Can you work these out from the model? Positions are in its coordinate system, mm. Face numbers are marked on the shaded views. A direction names the side the tool comes from. Give positions to 0.01 mm unless a question says otherwise; leave off trailing zeros. Order: outer loops, then holes, each group sorted by start corner. A loop starts at its lowest first (then second) coordinate and runs counter-clockwise, first axis right, second up.
Item 1: I want a section at D-D, the plane x = 125.5. Write out the boundary of the cut face in (y, z).
Item 2: I want a section at A-A, the plane y = -15. Write out the boundary of the cut face in (x, z).
Item 3: I'm going to push flat-ended pins straight in: pin 1 Ø8 at (x, y) = (112.5, 13.5) entering from +Z; pin 2 Ø10.5 at (x, z) = (144, 12) entering from +Y; pin 3 Ø1.5 at (y, z) = (-18, 6) entering from +X. Where does each tip first touch, or does it pass through?
Item 4: If we mould it in two halves opening along X, with no side actions, what happens to the marked faces 6, 7 and 8? For each: +X half, -X half, draft (parallel to the pull), parting line (faces both ways), or undercut.
Item 5: Which directions (+Z, -Z, +X, -X, +Y, -Y) give clear straight access to the entire face, cutting with the end or side of a thin tool? Please do the marked faces 1, 2, 3, 4 and 5.
Item 6: If I drill on line 1 along Y through (x, z) = (-1.5, -19); line 2 along Z through (x, y) = (0, 17.75); line 3 along X through (y, z) = (15.5, 10.5), over which ranges is the centre line in solid material (lowest first)?
Item 7: I want a section at B-B, the plane x = 2. Write out the boundary of the cut face in (y, z), then the cut area to 3 significant figures.
Item 8: I want a section at C-C, the plane y = 18.5. Write out the boundary of the cut face in (x, z), then the cut area to 3 significant figures.
```python
from build123d import *

# Parameters (mm, degrees)
F1_DEPTH      = 30.1625
F1_DEPTH_BACK = 30.1625
F2_DEPTH      = 11.1125
F2_DEPTH_BACK = 30.1625
F0_R          = 12.7
F3_DEPTH      = 30.1625
F3_DEPTH_BACK = 30.1625
F4_W          = 41.275
F4_H          = 34.798
F5_DEPTH      = 38.1
F6_W          = 11.1633
F6_H          = 50.8
F7_DEPTH      = 25.4
F7_DEPTH_BACK = 25.4
F8_R          = 6.35
F9_DEPTH      = 25.4
F10_R         = 7.874
F11_R         = 5.08
F12_F1_R      = 3.302
F12_F2_R      = 3.302


with BuildPart() as f1:
    # F0 (on Front) → F1 (new body, two sides)
    with BuildSketch(Plane.XZ) as f1_sk:
        with BuildLine():
            ThreePointArc((131.0386, 34.798), (127.4644153616, 16.0823576341), (117.2464, 0))
            Line((117.2464, 0), (117.2464, -22.352))
            Line((117.2464, -22.352), (194.2084, -22.352))
            Line((194.2084, -22.352), (194.2084, 0))
            Line((194.2084, 0), (150.0886, 0))
            Line((150.0886, 0), (150.0886, 34.798))
            Line((150.0886, 34.798), (131.0386, 34.798))
        make_face()
    extrude(amount=-F1_DEPTH)
    extrude(f1_sk.sketch, amount=F1_DEPTH_BACK)

    # F0 (on Front) → F2 (join, two sides)
    with BuildSketch(Plane.XZ) as f2_sk:
        Polygon((117.2464, 0), (85.852, 0), (91.8464, -22.352), (117.2464, -22.352), align=None)
    extrude(amount=F2_DEPTH)
    extrude(f2_sk.sketch, amount=-F2_DEPTH_BACK)

    # F0 (on Front) → F3 (join, two sides)
    with BuildSketch(Plane.XZ) as f3_sk:
        with BuildLine():
            Line((85.852, 0), (22.352, 0))
            ThreePointArc((22.352, 0), (15.8052507731, -15.8052507731), (0, -22.352))
            Line((0, -22.352), (91.8464, -22.352))
            Line((91.8464, -22.352), (85.852, 0))
        make_face()
        with BuildLine():
            ThreePointArc((0, -22.352), (15.8052507731, -15.8052507731), (22.352, 0))
            ThreePointArc((22.352, 0), (-15.8052507731, 15.8052507731), (0, -22.352))
        make_face()
        Circle(F0_R, mode=Mode.SUBTRACT)
    extrude(amount=F3_DEPTH)
    extrude(f3_sk.sketch, amount=-F3_DEPTH_BACK)

    # F4 (on face) → F5 (cut)
    with BuildSketch(Plane.YZ.offset(150.0886)):
        with Locations((9.525, 17.399)):
            Rectangle(F4_W, F4_H)
    extrude(amount=-F5_DEPTH, mode=Mode.SUBTRACT)

    # F6 (on Right) → F7 (cut, two sides)
    with BuildSketch(Plane.YZ) as f7_sk:
        with Locations((5.58165, 25.4)):
            Rectangle(F6_W, F6_H)
        with Locations((-5.58165, 25.4)):
            Rectangle(F6_W, F6_H)
        Polygon((11.1633, 0), (0, 0), (-11.1633, 0), (-11.1633, -23.6136056483), (11.1633, -23.6136056483), align=None)
    extrude(amount=-F7_DEPTH, mode=Mode.SUBTRACT)
    extrude(f7_sk.sketch, amount=F7_DEPTH_BACK, mode=Mode.SUBTRACT)

    # F8 (on face) → F9 (cut)
    with BuildSketch(Plane.XY):
        with Locations((155.3464, 7.8105)):
            Circle(F8_R)
    extrude(amount=-F9_DEPTH, mode=Mode.SUBTRACT)

    # F10
    f10_edges = [f1.edges().sort_by_distance(p)[0] for p in [
        (194.2084, 0, 0),
    ]]
    fillet(f10_edges, radius=F10_R)

    # F11
    f11_edges = [f1.edges().sort_by_distance(p)[0] for p in [
        (150.0886, -20.6375, 34.798),
    ]]
    fillet(f11_edges, radius=F11_R)

    # F12: fillet of radius 3.302 on 3 edges, made by hand

    # F12_f1
    f12_f1_edges = [f1.edges().sort_by_distance(p)[0] for p in [
        (150.0886, -20.6375, 0),
    ]]
    fillet(f12_f1_edges, radius=F12_F1_R)

    # F12_f2
    f12_f2_edges = [f1.edges().sort_by_distance(p)[0] for p in [
        (22.352, 20.6629, 0),
    ]]
    fillet(f12_f2_edges, radius=F12_F2_R)


solid = f1.part
```
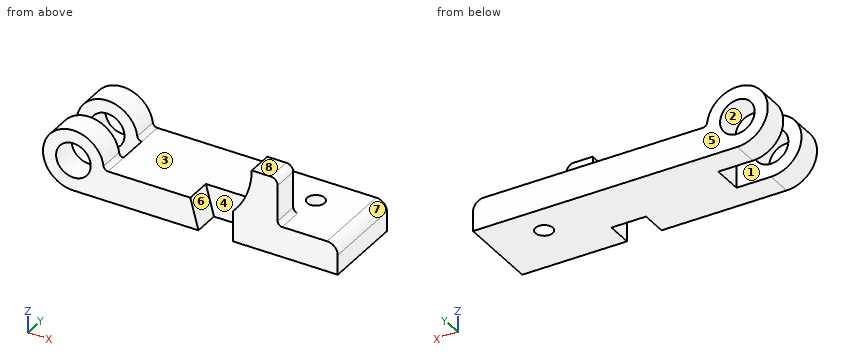
Results list:
1. outline: (-30.16, -22.35) - (30.16, -22.35) - (30.16, 0) - (-11.11, 0) - (-11.11, 11.73) - (-30.16, 11.73) - close
2. outline: (0, -22.35) - (91.85, -22.35) - (85.85, 0) - (25.44, 0) arc R3.3 cw to (22.17, 2.88) arc R22.35 ccw (long way) to start; (117.25, -22.35) - (194.21, -22.35) - (194.21, -7.87) arc R7.87 ccw to (186.33, 0) - (153.39, 0) arc R3.3 cw to (150.09, 3.3) - (150.09, 29.72) arc R5.08 ccw to (145.01, 34.8) - (131.04, 34.8) arc R50.8 cw to (117.25, 0) - close; hole circle Ø25.4 at (0, 0)
3. pin 1: stops at z = 0
3. pin 2: stops at y = -11.11
3. pin 3: stops at x = 150.09
4. face 6: undercut
4. face 7: +X half
4. face 8: draft
5. face 1: +Z, -Z, -X
5. face 2: +Y, -Y
5. face 3: +Z, +Y
5. face 4: +Z, -Y
5. face 5: +Z, -Z, +X, -X, +Y
6. line 1: y = -30.16 to -11.16, 11.16 to 30.16
6. line 2: z = -22.35 to -12.7, 12.7 to 22.35
6. line 3: x = -19.73 to -7.14, 7.14 to 19.73
7. outline: (-30.16, -22.35) - (-11.16, -22.35) - (-11.16, -12.54) - (-30.16, -12.54) - close; (-30.16, 12.54) - (-11.16, 12.54) - (-11.16, 22.26) - (-30.16, 22.26) - close; (11.16, -22.35) - (30.16, -22.35) - (30.16, -12.54) - (11.16, -12.54) - close; (11.16, 12.54) - (30.16, 12.54) - (30.16, 22.26) - (11.16, 22.26) - close
7. area: 742 mm2
8. outline: (0, -22.35) - (194.21, -22.35) - (194.21, -7.87) arc R7.87 ccw to (186.33, 0) - (25.44, 0) arc R3.3 cw to (22.17, 2.88) arc R22.35 ccw (long way) to start; hole circle Ø25.4 at (0, 0)
8. area: 5,000 mm2
